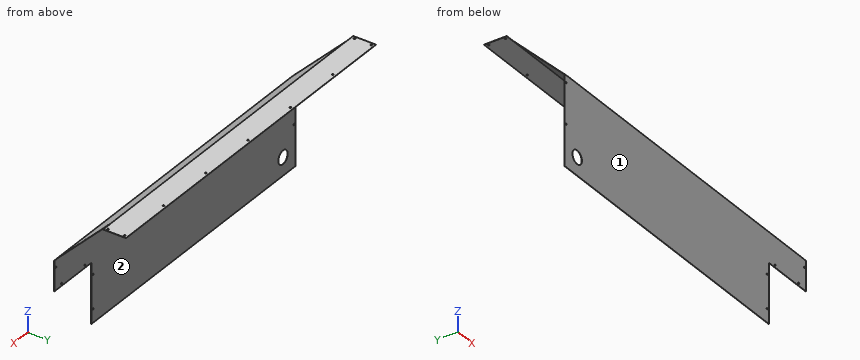
```python
from build123d import *

# Parameters (mm, degrees)
SM_BASE_FLANGE_1_DEPTH = 797
SKETCH_3_W             = 240.030004828
SKETCH_3_H             = 245.89814066
CUT_EXTRUDE_1_DEPTH    = 46
SKETCH_4_W             = 434.416474362
SKETCH_4_H             = 72.764759455
CUT_EXTRUDE_2_DEPTH    = 27.5
SKETCH_6_W             = 323.282059801
SKETCH_6_H             = 316.328682171
CUT_EXTRUDE_3_DEPTH    = 1076.72022385
SKETCH_7_R             = 3.5
CUT_EXTRUDE_4_DEPTH    = 1076.443164468
SKETCH_8_R             = 3.5
CUT_EXTRUDE_5_DEPTH    = 1076.72022385
SKETCH_10_R            = 3.5
CUT_EXTRUDE_6_DEPTH    = 976.892146686
SKETCH_11_R            = 3.5
CUT_EXTRUDE_7_DEPTH    = 977.427672693
SKETCH_12_R            = 30
CUT_EXTRUDE_8_DEPTH    = 1076.72022385


# Sheet-metal steps are written as plain solids
with BuildPart() as part:
    # Sketch 1 → 基体-法兰1 (new, symmetric)
    with BuildSketch(Plane(origin=(0, 0, 0), x_dir=(0, 0, -1), z_dir=(1, 0, 0))):
        with BuildLine():
            Line((0, 340), (0, 238.621320344))
            ThreePointArc((0, 238.621320344), (0.114180701, 238.047295195), (0.439339828, 237.560660172))
            Line((0.439339828, 237.560660172), (237.560660172, 0.439339828))
            ThreePointArc((237.560660172, 0.439339828), (238.047295195, 0.114180701), (238.621320344, 0))
            Line((238.621320344, 0), (638, 0))
            Line((638, 0), (638, 1))
            Line((638, 1), (238.621320344, 1))
            ThreePointArc((238.621320344, 1), (238.429978627, 1.038060234), (238.267766953, 1.146446609))
            Line((238.267766953, 1.146446609), (1.146446609, 238.267766953))
            ThreePointArc((1.146446609, 238.267766953), (1.038060234, 238.429978627), (1, 238.621320344))
            Line((1, 238.621320344), (1, 340))
            Line((1, 340), (0, 340))
        make_face()
    extrude(amount=SM_BASE_FLANGE_1_DEPTH, both=True)

    # 草图3 → 切除-拉伸1 (cut)
    with BuildSketch(Plane(origin=(797, 0, 0), x_dir=(0, 0, -1), z_dir=(1, 0, 0))):
        with Locations((118.60631793, 115.672250014)):
            Rectangle(SKETCH_3_W, SKETCH_3_H)
    cut_extrude_1 = extrude(amount=-CUT_EXTRUDE_1_DEPTH, mode=Mode.SUBTRACT)

    # 草图4 → 切除-拉伸2 (cut)
    with BuildSketch(Plane(origin=(797, 0, 0), x_dir=(0, 0, -1), z_dir=(1, 0, 0))):
        with Locations((445.827818623, 0.227200405)):
            Rectangle(SKETCH_4_W, SKETCH_4_H)
    cut_extrude_2 = extrude(amount=-CUT_EXTRUDE_2_DEPTH, mode=Mode.SUBTRACT)

    # 镜向2: 切除-拉伸1, 切除-拉伸2 across plane
    add(cut_extrude_1.mirror(Plane(origin=(0, 0, 0), x_dir=(0, 0, 1), z_dir=(1, 0, 0))), mode=Mode.SUBTRACT)
    add(cut_extrude_2.mirror(Plane(origin=(0, 0, 0), x_dir=(0, 0, 1), z_dir=(1, 0, 0))), mode=Mode.SUBTRACT)

    # 草图6 → 切除-拉伸3 (cut, through all)
    with BuildSketch(Plane(origin=(0, 1, 0), x_dir=(1, 0, 0), z_dir=(0, 1, 0))):
        with Locations((694.141029901, 530.164341086)):
            Rectangle(SKETCH_6_W, SKETCH_6_H)
    extrude(amount=-CUT_EXTRUDE_3_DEPTH, mode=Mode.SUBTRACT)

    # 草图7 → 切除-拉伸4 (cut, through all)
    with BuildSketch(Plane(origin=(0, 0, -1), x_dir=(-1, 0, 0), z_dir=(0, 0, -1))):
        with Locations(Location((0, 327, 0), (0, 0, 90))):
            Circle(SKETCH_7_R)
        with Locations(Location((270, 327, 0), (0, 0, 90))):
            Circle(SKETCH_7_R)
        with Locations(Location((540, 327, 0), (0, 0, 90))):
            Circle(SKETCH_7_R)
        with Locations(Location((786, 327, 0), (0, 0, 90))):
            Circle(SKETCH_7_R)
        with Locations(Location((786, 252, 0), (0, 0, 90))):
            Circle(SKETCH_7_R)
        with Locations(Location((-270, 327, 0), (0, 0, 90))):
            Circle(SKETCH_7_R)
        with Locations(Location((-540, 327, 0), (0, 0, 90))):
            Circle(SKETCH_7_R)
        with Locations(Location((-786, 327, 0), (0, 0, 90))):
            Circle(SKETCH_7_R)
        with Locations(Location((-786, 252, 0), (0, 0, 90))):
            Circle(SKETCH_7_R)
    extrude(amount=-CUT_EXTRUDE_4_DEPTH, mode=Mode.SUBTRACT)

    # 草图8 → 切除-拉伸5 (cut, through all)
    with BuildSketch(Plane(origin=(0, 1, 0), x_dir=(1, 0, 0), z_dir=(0, 1, 0))):
        with Locations(Location((-760, 452, 0), (0, 0, 270))):
            Circle(SKETCH_8_R)
        with Locations(Location((-760, 272, 0), (0, 0, 270))):
            Circle(SKETCH_8_R)
        with Locations(Location((521.5, 578, 0), (0, 0, 270))):
            Circle(SKETCH_8_R)
        with Locations(Location((521.5, 428, 0), (0, 0, 270))):
            Circle(SKETCH_8_R)
        with Locations(Location((573.5, 361, 0), (0, 0, 270))):
            Circle(SKETCH_8_R)
        with Locations(Location((723.5, 361, 0), (0, 0, 270))):
            Circle(SKETCH_8_R)
        with Locations(Location((760, 272, 0), (0, 0, 270))):
            Circle(SKETCH_8_R)
    extrude(amount=-CUT_EXTRUDE_5_DEPTH, mode=Mode.SUBTRACT)

    # 草图10 → 切除-拉伸6 (cut, through all)
    with BuildSketch(Plane(origin=(0, 119.707106781, -119.707106781), x_dir=(1, 0, 0), z_dir=(0, 0.7071067811865477, -0.7071067811865475))):
        with Locations(Location((740, 2.995728589, 0), (0, 0, 270))):
            Circle(SKETCH_10_R)
        with Locations(Location((740, -142.004271411, 0), (0, 0, 270))):
            Circle(SKETCH_10_R)
        with Locations(Location((740, 147.995728589, 0), (0, 0, 270))):
            Circle(SKETCH_10_R)
    extrude(amount=-CUT_EXTRUDE_6_DEPTH, mode=Mode.SUBTRACT)

    # 草图11 → 切除-拉伸7 (cut, through all)
    with BuildSketch(Plane(origin=(0, 119, -119), x_dir=(1, 0, 0), z_dir=(0, -0.7071067811865477, 0.7071067811865475))):
        with Locations(Location((-740, 142.004271411, 0), (0, 0, 270))):
            Circle(SKETCH_11_R)
        with Locations(Location((-740, -2.995728589, 0), (0, 0, 270))):
            Circle(SKETCH_11_R)
        with Locations(Location((-740, -147.995728589, 0), (0, 0, 270))):
            Circle(SKETCH_11_R)
    extrude(amount=-CUT_EXTRUDE_7_DEPTH, mode=Mode.SUBTRACT)

    # 草图12 → 切除-拉伸8 (cut, through all)
    with BuildSketch(Plane(origin=(0, 1, 0), x_dir=(-1, 0, 0), z_dir=(0, 1, 0))):
        with Locations(Location((689.5, -558, 0), (0, 0, 90))):
            Circle(SKETCH_12_R)
    extrude(amount=-CUT_EXTRUDE_8_DEPTH, mode=Mode.SUBTRACT)


solid = part.part
```
Input: part model. Units: mm. Frame: model coordinates. Face numbers are marked on the shaded views. A direction names the side the tool comes from. Give positions to 0.01 mm unless a question says otherwise; leave off trailing zeros. Loops run counter-clockwise (first coordinate to the right, second up) from the corner with the lowest first, then second, coordinate; pieces in that order, holes last. Notation, with made-up numbers: (40.5, 25.25) -> (96.5, 25.25) arc R13 cw to (96.5, 31.25) -> close; hole circle Ø10 at (19.5, -28). An arc over 180 degrees is marked (long way). Use a Markdown table: item, result.
Q1. Section query A-A, the plane z = -558. Return the cut outline in (x, y).
Entries:
| item | result |
|---|---|
| outline | (-769.5, 0) -> (-719.5, 0) -> (-719.5, 1) -> (-769.5, 1) -> close; (-659.5, 0) -> (532.5, 0) -> (532.5, 1) -> (-659.5, 1) -> close |
Q2. Section query C-C, the plane z = -76.5. Return the cut outline in (x, y), plus the area to 3 significant figures.
Entries:
| item | result |
|---|---|
| outline | (-751, 161.5) -> (751, 161.5) -> (751, 162.91) -> (-751, 162.91) -> close |
| area | 2,120 mm² |
Q3. Section query D-D, the plane y = 84.5. Return the cut outline in (x, z), plus the area to 3 significant figures.
Entries:
| item | result |
|---|---|
| outline | (-751, -154.91) -> (751, -154.91) -> (751, -153.5) -> (-751, -153.5) -> close |
| area | 2,120 mm² |
Q4. Section query B-B, the plane x = -140.5. Return the cut outline in (y, z), plus the area to 3 significant figures.
Entries:
| item | result |
|---|---|
| outline | (0, -638) -> (1, -638) -> (1, -238.62) arc R0.5 cw to (1.15, -238.27) -> (238.27, -1.15) arc R0.5 cw to (238.62, -1) -> (340, -1) -> (340, 0) -> (238.62, 0) arc R1.5 ccw to (237.56, -0.44) -> (0.44, -237.56) arc R1.5 ccw to (0, -238.62) -> close |
| area | 838 mm² |
Q5. First-contact query: P1, Ø11, axis at x = -786, y = 252, coming from the -Z side; P2, Ø1.1, axis at y = 0.5, z = -536, coming from the -X side; P3, Ø4, axis at x = -432, y = 179.5, coming from the +Z side; P4, Ø5.5, axis at x = -270, y = 327, coming from the +Z side. Flat tips, straight axial feed; report the tip coordinate or a pass-through.
Entries:
| item | result |
|---|---|
| P1 | stops at z = -1 |
| P2 | stops at x = -769.5 |
| P3 | stops at z = -56.5 |
| P4 | passes through |
Q6. Ray query, probe 1 along X at (y, z) = (252, -0.2); probe 2 along Z at (x, y) = (521.5, 0.7); probe 3 along X at (y, z) = (0.3, -361). Return the intervals inside material, ascending. Write a range as from..to.
Entries:
| item | result |
|---|---|
| probe 1 | x = -797..-789.5, -782.5..782.5, 789.5..797 |
| probe 2 | z = -638..-581.5, -574.5..-431.5, -424.5..-237.3 |
| probe 3 | x = -769.5..570, 577..720, 727..769.5 |
Q7. Access query for the marked faces 1 and 2. Directions: +Z, -Z, +X, -X, +Y, -Y. A direction counts if a zero-diameter tool reaches every point of the face in a straight line with its end or side. Return the directions, or none.
Entries:
| item | result |
|---|---|
| face 1 | +Z, -Z, +X, -X, -Y |
| face 2 | -Z, +X, -X, +Y |
